Autodesk Inventor part; units mm, degrees
ref_plane "YZ Plane" through (0, 0, 0) normal (1, 0, 0) x (0, 1, 0)
ref_plane "XZ Plane" through (0, 0, 0) normal (0, 1, 0) x (-1, 0, 0)
ref_plane "XY Plane" through (0, 0, 0) normal (0, 0, 1) x (1, 0, 0)
sketch "Sketch1" plane through (0, 0, 0) normal (0, 0, 1) x (1, 0, 0)
  circle A0 centre (0, 0) radius 47.625
  dimension "d0" = 95.25
extrude "Extrusion1" add sketch "Sketch1" along normal blind 3.175
sketch "Sketch3" plane through (0, 0, 3.175) normal (0, 0, 1) x (1, 0, 0)
  line L0 (1.27, 9.525) -> (20.32, 9.525)
  line L1 (20.32, 9.525) -> (20.32, 0)
  line L2 (20.32, 0) -> (1.27, 0)
  line L3 (1.27, 0) -> (1.27, 9.525)
  line L4 (0, 0) -> (0, -11.0035)
  line L5 (-1.27, 9.525) -> (-20.32, 9.525)
  line L6 (-20.32, 9.525) -> (-20.32, 0)
  line L7 (-20.32, 0) -> (-1.27, 0)
  line L8 (-1.27, 0) -> (-1.27, 9.525)
  dimension "d11" = 19.05
  dimension "d12" = 9.525
  dimension "d13" = 1.27
  dimension "d14" = 0
extrude "Extrusion3" add sketch "Sketch3" along normal blind 6.604
sketch "Sketch4" plane through (1.27, 9.525, 3.175) normal (0, 1, 0) x (1, 0, 0)
  circle A0 centre (4.445, -2.794) radius 1.397
  line L0 (19.05, -6.604) -> (0, -6.604)
  circle A1 centre (14.605, -2.794) radius 1.397
  line L1 (9.525, -6.604) -> (9.525, -7.9119)
  line L2 (-1.27, 3.175) -> (-1.27, 8.3959)
  circle A2 centre (-6.985, -2.794) radius 1.397
  circle A3 centre (-17.145, -2.794) radius 1.397
  dimension "d17" = 2.794
  dimension "d18" = 3.81
  dimension "d19" = 2.794
  dimension "d20" = 3.81
  dimension "d21" = 10.16
  dimension "d22" = 5.08
extrude "Extrusion4" cut sketch "Sketch4" against normal through all
sketch "Sketch5" plane through (0, 0, 3.175) normal (0, 0, 1) x (1, 0, 0)
  circle A0 centre (20.795, 25.8191) radius 3.175
  line L0 (0, 0) -> (0, 16.9345)
  circle A1 centre (-20.795, 25.8191) radius 3.175
  dimension "d25" = 6.35
  dimension "d26" = 20.795
  dimension "d27" = 25.8191
extrude "Extrusion5" cut sketch "Sketch5" against normal blind 25.4
sketch "Sketch6" plane through (0, 0, 3.175) normal (0, 0, 1) x (1, 0, 0)
  line L0 (0, 0) -> (0, 41.91)
  circle A0 centre (0, 41.91) radius 1.8415
  circle A1 centre (-36.2951, 20.955) radius 1.8415
  circle A2 centre (-36.2951, -20.955) radius 1.8415
  circle A3 centre (0, -41.91) radius 1.8415
  circle A4 centre (36.2951, -20.955) radius 1.8415
  circle A5 centre (36.2951, 20.955) radius 1.8415
  dimension "d30" = 41.91
  dimension "d31" = 3.683
  dimension "d34" = 360
extrude "Extrusion6" cut sketch "Sketch6" against normal blind 25.4
sketch "Sketch9" plane through (0, 0, 3.175) normal (0, 0, 1) x (1, 0, 0)
  circle A0 centre (0, 0) radius 36.322
  line L0 (-1.27, 9.525) -> (-20.32, 9.525)
  line L1 (-20.32, 9.525) -> (-20.32, 0)
  line L2 (-20.32, 0) -> (-1.27, 0)
  line L3 (-1.27, 0) -> (-1.27, 9.525)
  line L4 (20.32, 9.525) -> (1.27, 9.525)
  line L5 (1.27, 9.525) -> (1.27, 0)
  line L6 (1.27, 0) -> (20.32, 0)
  line L7 (20.32, 0) -> (20.32, 9.525)
  line L8 (-20.32, 0) -> (-20.32, 9.525)
  line L9 (-20.32, 9.525) -> (-35.0508, 9.525)
  line L10 (-20.32, 0) -> (-36.322, 0)
  line L11 (-1.27, 9.525) -> (-1.27, 0)
  line L12 (1.27, 9.525) -> (1.27, 0)
  line L13 (-1.27, 9.525) -> (1.27, 9.525)
  line L14 (-1.27, 0) -> (1.27, 0)
  line L15 (20.32, 0) -> (36.322, 0)
  line L16 (20.32, 9.525) -> (35.0508, 9.525)
  point P0 (-28.956, -21.928)
  point P1 (-20.701, -29.8455)
  point P2 (28.956, -21.928)
extrude "Extrusion9" cut sketch "Sketch9" against normal through all contours A0 L10 L2 L14 L6 L15 | L16 L4 L13 L0 L9 A0
sketch "Sketch10" plane through (-1.27, 9.525, 3.175) normal (0, 1, 0) x (1, 0, 0)
  line L0 (0, 0) -> (0, -6.604)
  line L1 (2.54, 0) -> (2.54, -6.604)
  line L2 (0, -6.604) -> (2.54, -6.604)
  line L3 (2.54, -6.604) -> (2.54, 0)
  line L4 (2.54, 0) -> (0, 0)
  line L5 (0, 0) -> (0, -6.604)
  point P0 (1.27, 3.175)
extrude "Extrusion10" add sketch "Sketch10" against normal up to surface (9.525 mm away)
chamfer "Chamfer1" distance 6.35 distance2 3.175 1 edges at (20.32, 4.7625, 3.175) measured on face at (-30.5643, 3.175, 3.175)
chamfer "Chamfer2" distance 6.35 distance2 3.175 1 edges at (-20.32, 4.7625, 3.175) measured on face at (-30.5643, 3.175, 3.175)
fillet "Fillet3" radius 3.175 4 edges at (-35.0508, 9.525, 1.5875) (-36.322, 0, 1.5875) (35.0508, 9.525, 1.5875) (36.322, 0, 1.5875)
properties part number "rearServoAttachmentPlate" material "ABS Plastic"
Geometry check sheet. Reference: the model listing, model coordinates, mm. A direction names the side the tool comes from. Round coordinates to 2 decimals unless told otherwise and drop trailing zeros. Order: outer loops, then holes, each group sorted by start corner. A loop starts at its lowest first (then second) coordinate and runs counter-clockwise, first axis right, second up. Notation, with made-up numbers: M 57.5,-4.75 L 112.5,-4.75 A14 cw 112.5,12.25 Z; hole C 77.5,79.25 d7. An arc over 180 degrees is marked long. Write item = value, one per line.
Q1. Set-up check for faces 1 (the flat face through (20.32, 5, 8)), 2 (the cylindrical face through (-0.75, -36.314, 1.61)), 3 (the flat face through (-20.32, 5, 8)): record each of +Z, -Z, +X, -X, +Y, -Y from which the full face is reachable in a straight line by a thin tool's end or side.
Answer block:
face_1 = +Z, +X, +Y, -Y
face_2 = +Z, -Z
face_3 = +Z, -X, +Y, -Y
Q2. Depth check by flat-ended pin: pin 1 Ø3.5 at (x, z) = (-5.715, 5.969) entering from -Y; pin 2 Ø5 at (x, y) = (-36.3, -20.96) entering from +Z (3 decimals); pin 3 Ø6 at (x, y) = (36.3, 20.96) entering from -Z; pin 4 Ø1 at (y, z) = (5.5, 7.5) entering from -X. Enter the tip coordinate at first touch or a pass-through.
Answer block:
pin_1 = 0
pin_2 = 3.175
pin_3 = 0
pin_4 = -20.32
Q3. Section check B-B (y = -18). Enter the section's corners in (x, z) (3 decimals).
Answer block:
outline = M -44.092,0 L -31.548,0 L -31.548,3.175 L -44.092,3.175 Z; M 31.548,0 L 44.092,0 L 44.092,3.175 L 31.548,3.175 Z
Q4. Section check A-A (x = 0). Enter the section's corners in (y, z) (1 decimal), plus the area to 3 significant figures.
Answer block:
outline = M -47.6,0 L -43.8,0 L -43.8,3.2 L -47.6,3.2 Z; M -40.1,0 L -36.3,0 L -36.3,3.2 L -40.1,3.2 Z; M 0,0 L 9.5,0 L 9.5,9.8 L 0,9.8 Z; M 36.3,0 L 40.1,0 L 40.1,3.2 L 36.3,3.2 Z; M 43.8,0 L 47.6,0 L 47.6,3.2 L 43.8,3.2 Z
area = 142 mm^2
Q5. Section check C-C (x = 10.5). Enter the section's corners in (y, z) (3 decimals), plus the area to 3 significant figures.
Answer block:
outline = M -46.453,0 L -34.771,0 L -34.771,3.175 L -46.453,3.175 Z; M 0,0 L 9.525,0 L 9.525,9.779 L 0,9.779 Z; M 34.771,0 L 46.453,0 L 46.453,3.175 L 34.771,3.175 Z
area = 167 mm^2
Q6. Scan lines: line 1 (Y direction, x = 0, z = 1.9) (1 decimal); line 2 (X direction, y = 3, z = 6.75); line 3 (X direction, y = 6, z = 4.75). Record each from-to range of solid material in increasing order.
Answer block:
line_1 = -47.6 to -43.8, -40.1 to -36.3, 0 to 9.5, 36.3 to 40.1, 43.8 to 47.6
line_2 = -20.32 to -17.03, -14.72 to -6.87, -4.56 to 4.56, 6.87 to 14.72, 17.03 to 20.32
line_3 = -23.52 to -16.56, -15.19 to -6.4, -5.03 to 5.03, 6.4 to 15.19, 16.56 to 23.52
Q7. Section check D-D (y = 41.91). Enter the section's corners in (x, z) (1 decimal).
Answer block:
outline = M -22.6,0 L -1.8,0 L -1.8,3.2 L -22.6,3.2 Z; M 1.8,0 L 22.6,0 L 22.6,3.2 L 1.8,3.2 Z
Q8. Release check for a two-part mould opening along Y. For faces 4 (the cylindrical face through (-37.794, 28.979, 1.565)), 5 (the cylindrical face through (35.32, -1.013, 1.565)), 6 (the flat face through (-28.4, 0.2, 3.175)) record: released by +Y, released by -Y, zero draft, split by the parting line, or undercut.
Answer block:
face_4 = split by the parting line
face_5 = undercut
face_6 = zero draft
